Build history of the part. All positions in model axes, mm. A direction names the side the tool comes from. Give positions to 0.01 mm unless a question says otherwise; leave off trailing zeros. Order: outer loops, then holes, each group sorted by start corner. A loop starts at its lowest first (then second) coordinate and runs counter-clockwise, first axis right, second up. Notation, with made-up numbers: M -2.5,55 L 15.5,55 A15 ccw 15.5,76 Z; hole C -16,-8.75 d7. An arc over 180 degrees is marked long. One line per item, written item: value. Start each with the question number.
from build123d import *

# Parameters (mm, degrees)
ESQUISSE1_R        = 2.5
ESQUISSE1_W        = 134
ESQUISSE1_H        = 10
BOSS_EXTRU_2_DEPTH = 10
ESQUISSE1_26_W     = 20
ESQUISSE1_26_H     = 2
BOSS_EXTRU_3_DEPTH = 2
ESQUISSE1_27_R     = 2.5
BOSS_EXTRU_4_DEPTH = 15
ESQUISSE1_28_W     = 4.5
ESQUISSE1_28_H     = 2.5
BOSS_EXTRU_5_DEPTH = 10
CONG_1_R           = 1
CONG_2_R           = 1
CONG_3_R           = 1
CONG_4_R           = 2
CONG_5_R           = 2


with BuildPart() as part:
    # Esquisse1 → Boss.-Extru.2 (new body)
    # profile 1 of 7: a face of its own
    with BuildSketch(Plane.XY):
        Polygon((-151.59444934, 48.560080763), (-151.59444934, 38.560080763), (-143.805852374, 38.560080763), (-123.805852374, 38.560080763), (-17.59444934, 38.560080763), (-17.59444934, 42.310080763), (-17.59444934, 44.810080763), (-17.59444934, 48.560080763), align=None)
        with Locations((-84.59444934, 43.560080763)):
            Circle(ESQUISSE1_R, mode=Mode.SUBTRACT)
    # profile 2 of 7: a face of its own
    with BuildSketch(Plane.XY):
        Polygon((-191.59444934, 38.560080763), (-151.59444934, 38.560080763), (-151.59444934, 48.560080763), (-191.59444934, 44.060080763), align=None)
    # profile 3 of 7: a face of its own
    with BuildSketch(Plane.XY):
        with BuildLine():
            ThreePointArc((-191.59444934, -101.939919237), (-208.258682651, -33.939919237), (-191.59444934, 34.060080763))
            Line((-191.59444934, 34.060080763), (-191.59444934, 38.560080763))
            Line((-191.59444934, 38.560080763), (-191.59444934, 44.060080763))
            ThreePointArc((-191.59444934, 44.060080763), (-217.658663565, -33.939919237), (-191.59444934, -111.939919237))
            Line((-191.59444934, -111.939919237), (-191.59444934, -106.439919237))
            Line((-191.59444934, -106.439919237), (-191.59444934, -101.939919237))
        make_face()
        with Locations((-214.593861295, -36.363237388)):
            Circle(ESQUISSE1_R, mode=Mode.SUBTRACT)
    # profile 4 of 7: a face of its own
    with BuildSketch(Plane.XY):
        Polygon((-191.59444934, 38.560080763), (-191.59444934, 34.060080763), (-151.59444934, 38.560080763), align=None)
    # profile 5 of 7: a face of its own
    with BuildSketch(Plane.XY):
        Polygon((-191.59444934, -111.939919237), (-191.59444934, -106.439919237), (-151.59444934, -106.439919237), (-151.59444934, -116.439919237), align=None)
    # profile 6 of 7: a face of its own
    with BuildSketch(Plane.XY):
        Polygon((-151.59444934, -106.439919237), (-191.59444934, -101.939919237), (-191.59444934, -106.439919237), align=None)
    # profile 7 of 7: a face of its own
    with BuildSketch(Plane.XY):
        with Locations((-84.59444934, -111.439919237)):
            Rectangle(ESQUISSE1_W, ESQUISSE1_H)
        with Locations((-84.59444934, -111.439919237)):
            Circle(ESQUISSE1_R, mode=Mode.SUBTRACT)
    extrude(amount=BOSS_EXTRU_2_DEPTH)

    # Esquisse1<26> → Boss.-Extru.3 (add)
    with BuildSketch(Plane.XY):
        with Locations((-133.805852374, -105.439919237)):
            Rectangle(ESQUISSE1_26_W, ESQUISSE1_26_H)
        with Locations((-133.805852374, 37.560080763)):
            Rectangle(ESQUISSE1_26_W, ESQUISSE1_26_H)
    extrude(amount=BOSS_EXTRU_3_DEPTH)

    # Esquisse1<27> → Boss.-Extru.4 (add)
    with BuildSketch(Plane.XY):
        with Locations((-214.593861295, -36.363237388)):
            Circle(ESQUISSE1_27_R)
        with Locations((-84.59444934, 43.560080763)):
            Circle(ESQUISSE1_27_R)
        with Locations((-84.59444934, -111.439919237)):
            Circle(ESQUISSE1_27_R)
    extrude(amount=BOSS_EXTRU_4_DEPTH)

    # Esquisse1<28> → Boss.-Extru.5 (add)
    with BuildSketch(Plane.XY):
        with Locations((-15.34444934, 43.560080763)):
            Rectangle(ESQUISSE1_28_W, ESQUISSE1_28_H)
        with Locations((-15.34444934, -111.439919237)):
            Rectangle(ESQUISSE1_28_W, ESQUISSE1_28_H)
    extrude(amount=BOSS_EXTRU_5_DEPTH)

    # Congé1
    cong_1_edges = [part.edges().sort_by_distance(p)[0] for p in [
        (-87.09444934, 43.560080763, 15),
    ]]
    fillet(cong_1_edges, radius=CONG_1_R)

    # Congé2
    cong_2_edges = [part.edges().sort_by_distance(p)[0] for p in [
        (-87.09444934, -111.439919237, 15),
    ]]
    fillet(cong_2_edges, radius=CONG_2_R)

    # Congé3
    cong_3_edges = [part.edges().sort_by_distance(p)[0] for p in [
        (-217.093861295, -36.363237388, 15),
    ]]
    fillet(cong_3_edges, radius=CONG_3_R)

    # Congé4
    cong_4_edges = [part.edges().sort_by_distance(p)[0] for p in [
        (-133.805852374, -104.439919237, 0),
    ]]
    fillet(cong_4_edges, radius=CONG_4_R - 0.0001)  # a hair under: the kernel refuses the full size

    # Congé5
    cong_5_edges = [part.edges().sort_by_distance(p)[0] for p in [
        (-133.805852374, 36.560080763, 0),
    ]]
    fillet(cong_5_edges, radius=CONG_5_R - 0.0001)  # a hair under: the kernel refuses the full size


solid = part.part
1) Drop flat-ended pins along their axis: P1, Ø1.3, axis at x = -15, z = 3.5, coming from the -Y side; P2, Ø4, axis at y = 47, z = 6, coming from the +X side; P3, Ø4, axis at y = -6, z = 3, coming from the -X side. Give the stop position or say it passes through.
2) Slice it at A-A (x = -200). List the corners of the cut face in (y, z).
3) Drill centre lines: line 1 (Y direction, x = -96.5, z = 4.5); line 2 (X direction, y = 12, z = 6.25); line 3 (Y direction, x = -155, z = 7). Where is each one in solid material? Low to high.
4) Slice it at C-C (y = -24.5). List the corners of the cut face in (x, z).
5) Tool access for faces 1 (the flat face through (-15, -110.19, 5)), 2 (the cylindrical face through (-85.14, -113.88, 11.97)), 3 (the flat face through (-15, 44.81, 5)): list every direction of +Z, -Z, +X, -X, +Y, -Y with a clear straight run to the whole face (end or side of a thin tool).
6) Slice it at D-D (x = -175). List the corners of the cut face in (y, z).
7) Slice it at B-B (z = 7.25). List the corners of the cut face in (x, y).
Results list:
1. P1: stops at y = -112.69
1. P2: stops at x = -17.59
1. P3: stops at x = -215.04
2. outline: M -99.29,0 L -82.53,0 L -82.53,10 L -99.29,10 Z; M 14.65,0 L 31.41,0 L 31.41,10 L 14.65,10 Z
3. line 1: y = -116.44 to -106.44, 38.56 to 48.56
3. line 2: x = -209.25 to -200.9
3. line 3: y = -116.06 to -106.06, 38.18 to 48.18
4. outline: M -217.31,0 L -207.96,0 L -207.96,10 L -217.31,10 Z
5. face 1: +Z, -Z, +X
5. face 2: +Z
5. face 3: +Z, -Z, +X, +Y
6. outline: M -113.81,0 L -103.81,0 L -103.81,10 L -113.81,10 Z; M 35.93,0 L 45.93,0 L 45.93,10 L 35.93,10 Z
7. outline: M -191.59,-111.94 L -151.59,-116.44 L -17.59,-116.44 L -17.59,-112.69 L -13.09,-112.69 L -13.09,-110.19 L -17.59,-110.19 L -17.59,-106.44 L -151.59,-106.44 L -191.59,-101.94 A147.07 cw -191.59,34.06 L -151.59,38.56 L -17.59,38.56 L -17.59,42.31 L -13.09,42.31 L -13.09,44.81 L -17.59,44.81 L -17.59,48.56 L -151.59,48.56 L -191.59,44.06 A129.74 ccw Z
